```python
from build123d import *

# Parameters (mm, degrees)
F1_DEPTH = 6.6
F2_W     = 12.675607577
F2_H     = 6.6
F3_DEPTH = 4


with BuildPart() as f1:
    # F0 (on Top) → F1 (new body)
    with BuildSketch(Plane.XY):
        with BuildLine():
            Line((7.45, 0), (4.65, 0))
            ThreePointArc((4.65, 0), (-3.2880465325, -3.2880465325), (0, 4.65))
            Line((0, 4.65), (0, 7.45))
            ThreePointArc((0, 7.45), (-5.2679455198, 5.2679455198), (-7.45, 0))
            ThreePointArc((-7.45, 0), (0, -7.45), (7.45, 0))
        make_face()
        with BuildLine():
            ThreePointArc((0, 4.65), (3.2880465325, 3.2880465325), (4.65, 0))
            Line((4.65, 0), (7.45, 0))
            ThreePointArc((7.45, 0), (5.2679455198, 5.2679455198), (0, 7.45))
            Line((0, 7.45), (0, 4.65))
        make_face()
        with BuildLine():
            ThreePointArc((0, 7.45), (5.2679455198, 5.2679455198), (7.45, 0))
            Line((7.45, 0), (27.8879404068, 0))
            Line((27.8879404068, 0), (27.8879404068, 7.45))
            Line((27.8879404068, 7.45), (0, 7.45))
        make_face()
        with BuildLine():
            ThreePointArc((-7.45, 0), (-5.2679455198, 5.2679455198), (0, 7.45))
            Line((0, 7.45), (-42.95, 7.45))
            Line((-42.95, 7.45), (-42.95, 0))
            Line((-42.95, 0), (-7.45, 0))
        make_face()
    extrude(amount=F1_DEPTH)

    # F2 (on face) → F3 (join)
    with BuildSketch(Plane(origin=(-42.95, 0, 0), x_dir=(0, -1, 0), z_dir=(-1, 0, 0))):
        with Locations((-6.3378037885, 3.3)):
            Rectangle(F2_W, F2_H)
    extrude(amount=F3_DEPTH)


solid = f1.part
```
Input: part model. Units: mm. Frame: model coordinates. A direction names the side the tool comes from. Give positions to 0.01 mm unless a question says otherwise; leave off trailing zeros. Loops run counter-clockwise (first coordinate to the right, second up) from the corner with the lowest first, then second, coordinate; pieces in that order, holes last. Notation, with made-up numbers: M -3,-15 L 56,-15 A27 ccw 56,7 Z; hole C 86,63 d7. An arc over 180 degrees is marked long. Answer as CSV lines item,"result". Start each with the question number.
1. Reachability of faces 1 (the face through (-9, 3, 0)), 2 (the face through (18, 0, 3)), 3 (the face through (-7, 7.45, 3)), 4 (the face through (-27, 0, 3)) from +Z, -Z, +X, -X, +Y, -Y: full face, straight path, thin tool, end or side. Return the list, or none.
2. Section A-A on z = 1.5. Return loops of the section in (x, y), plus the area to 3 significant figures.
3. Section C-C on x = 9.5. Return loops of the section in (y, z), plus the area to 3 significant figures.
4. Line query: L1, parallel to Y at x = 0, z = 4; L2, parallel to Y at x = 9, z = 4.5; L3, parallel to X at y = -4, z = 1.75. Output: solid intervals per line, ascending.
5. Pin query (flat end, axial travel): P1, Ø1, axis at x = -17, z = 4, coming from the +Y side; P2, Ø1, axis at x = 15.5, y = 9, coming from the +Z side; P3, Ø2.5, axis at y = 11.5, z = 3.5, coming from the +X side. Return the tip coordinate at first contact, or that it passes through.
6. Section D-D on y = 9.5. Return loops of the section in (x, z), plus the area to 3 significant figures.
7. Section B-B on y = 2. Return loops of the section in (x, z).
Computed values:
1,face 1,"-Z, +X, -X, +Y, -Y"
1,face 2,"+Z, -Z, +X, -Y"
1,face 3,"+Z, -Z, +X, +Y"
1,face 4,"+Z, -Z, -X, -Y"
2,outline,"M -46.95,0 L -7.45,0 A7.45 ccw 7.45,0 L 27.89,0 L 27.89,7.45 L -42.95,7.45 L -42.95,12.68 L -46.95,12.68 Z; hole C 0,0 d9.3"
2,area,"598 mm²"
3,outline,"M 0,0 L 7.45,0 L 7.45,6.6 L 0,6.6 Z"
3,area,"49.2 mm²"
4,L1,"y = -7.45 to -4.65, 4.65 to 7.45"
4,L2,"y = 0 to 7.45"
4,L3,"x = -6.29 to -2.37, 2.37 to 6.29"
5,P1,"stops at y = 7.45"
5,P2,"passes through"
5,P3,"stops at x = -42.95"
6,outline,"M -46.95,0 L -42.95,0 L -42.95,6.6 L -46.95,6.6 Z"
6,area,"26.4 mm²"
7,outline,"M -46.95,0 L -4.2,0 L -4.2,6.6 L -46.95,6.6 Z; M 4.2,0 L 27.89,0 L 27.89,6.6 L 4.2,6.6 Z"
